from build123d import *

# Parameters (mm, degrees)
F1_DEPTH    = 20
F2_START    = 18.5
F2_DEPTH    = 1.5
F3_START    = 17.5
F0_W        = 1.9191285201
F0_H        = 0.8
F3_DEPTH    = 2
F4_START    = 17.5
F0_H_2      = 0.9897637812
F4_DEPTH    = 2
F5_DEPTH    = 17.5
F6_DEPTH    = 18.5
F7_START    = 17.5
F0_W_2      = 35
F0_H_3      = 9.3263725303
F7_DEPTH    = 2.5
F8_T1_DEPTH = 40.1796577476
F8_T3_DEPTH = 14.5060302779


# Not quite as in the source:
# - a fillet or chamfer that OpenCascade refuses, or shapes differently, is made with other operations: its cross-section is extruded or revolved along the edge and cut away or added


with BuildPart() as f1:
    # F0 (on Top) → F1 (new body)
    with BuildSketch(Plane.XY):
        Polygon((-14.85, 2), (14.85, 2), (14.85, -1), (14.85, -2), (0.95956426, -2), (0.95956426, -2.8), (15.65, -2.8), (15.65, 2.8), (-15.65, 2.8), (-15.65, -2.8), (-0.95956426, -2.8), (-0.95956426, -2), (-14.85, -2), (-14.85, -1), align=None)
    extrude(amount=F1_DEPTH)

    # F0 (on Top) → F2 (join)
    with BuildSketch(Plane.XY.offset(F2_START)):
        Polygon((14.85, -2), (14.85, -1), (-14.85, -1), (-14.85, -2), (-0.95956426, -2), (-0.95956426, -1.4462094987), (0.4121778399, -1.4462094987), (0.95956426, -2), align=None)
    extrude(amount=F2_DEPTH)

    # F0 (on Top) → F3 (join)
    with BuildSketch(Plane.XY.offset(F3_START)):
        with Locations((0, -2.4)):
            Rectangle(F0_W, F0_H)
        Polygon((-0.95956426, -2), (0.95956426, -2), (0.4121778399, -1.4462094987), (-0.95956426, -1.4462094987), align=None)
    extrude(amount=F3_DEPTH)

    # F0 (on Top) → F4 (join)
    with BuildSketch(Plane.XY.offset(F4_START)):
        with Locations((0, -3.2948818906)):
            Rectangle(F0_W, F0_H_2)
    extrude(amount=F4_DEPTH)

    # F0 (on Top) → F5 (join)
    with BuildSketch(Plane.XY):
        with Locations((0, -2.4)):
            Rectangle(F0_W, F0_H)
    extrude(amount=F5_DEPTH)

    # F0 (on Top) → F6 (cut)
    with BuildSketch(Plane.XY):
        Polygon((-0.95956426, -2), (0.95956426, -2), (0.4121778399, -1.4462094987), (-0.95956426, -1.4462094987), align=None)
    extrude(amount=F6_DEPTH, mode=Mode.SUBTRACT)

    # F0 (on Top) → F7 (join)
    with BuildSketch(Plane.XY.offset(F7_START)):
        with Locations((0, 0.4131862652)):
            Rectangle(F0_W_2, F0_H_3)
        Polygon((15.65, -2.8), (0.95956426, -2.8), (0.95956426, -3.7897637812), (-0.95956426, -3.7897637812), (-0.95956426, -2.8), (-15.65, -2.8), (-15.65, 2.8), (15.65, 2.8), align=None, mode=Mode.SUBTRACT)
    extrude(amount=F7_DEPTH)

    # F8: chamfer of 0.5 x 1 on 4 edges, made by hand

    # F8_s2 → F8_t1 (cut)
    with BuildSketch(Plane.YZ.offset(-20.0898288738)):
        Polygon((4.0763725303, 20), (5.0763725303, 19.5), (5.0763725303, 20), align=None)
        Polygon((-3.25, 20), (-4.25, 19.5), (-4.25, 20), align=None)
    extrude(amount=F8_T1_DEPTH, mode=Mode.SUBTRACT)

    # F8_s4 → F8_t3 (cut)
    with BuildSketch(Plane.XZ.offset(-7.6662014041)):
        Polygon((-17.5, 19.5), (-16.5, 20), (-17.5, 20), align=None)
        Polygon((16.5, 20), (17.5, 19.5), (17.5, 20), align=None)
    extrude(amount=F8_T3_DEPTH, mode=Mode.SUBTRACT)


solid = f1.part
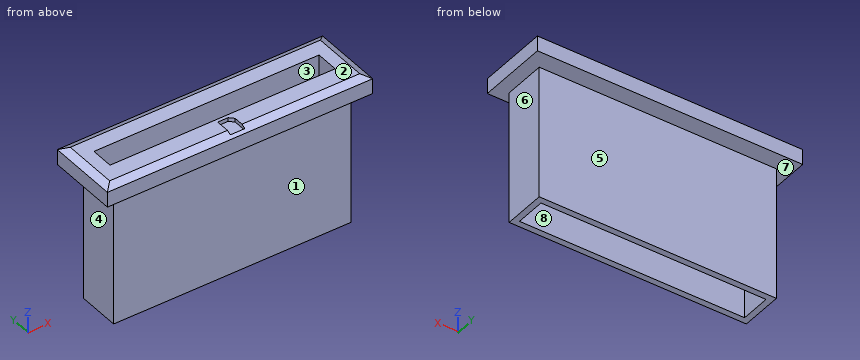
CAD build for the part. Positions are in the model's coordinates, mm. Face numbers are marked on the shaded views. A direction names the side the tool comes from. Round coordinates to 2 decimals unless told otherwise and drop trailing zeros. Write each loop counter-clockwise with the first axis right and the second up, starting at its lowest first coordinate (ties: lowest second). Pieces come first, ordered by that corner, then holes.
(1) Mould opens along X. For the marked faces 6, 7 and 8 say: pulls with the +X half, pulls with the -X half, needs draft (parallel to the pull), parting line crosses it, or undercut.
(2) Drop flat-ended pins along their axis: P1, Ø1.1, axis at x = -4.5, y = -1.5, coming from the -Z side; P2, Ø2, axis at y = 0, z = 12, coming from the +X side; P3, Ø1.5, axis at y = -3, z = 13.5, coming from the -X side; P4, Ø5.5, axis at x = 7, z = 6.5, coming from the +Y side. Give the stop position or say it passes through.
(3) 3-axis set-ups, long thin cutter, end or side, ignore diameter. For the marked faces 1, 2, 3, 4 and 5: which of +Z, -Z, +X, -X, +Y, -Y reach the whole face in a straight line?
(4) Slice it at C-C, the plane y = -0.5. Write the cut outline in (x, z).
(5) Slice it at B-B, the plane z = 6.5. Write the cut outline in (x, y), and give its area (3 significant figures).
(6) Slice it at A-A, the plane x = -0.5. Write the cut outline in (y, z).
(7) Probe line 1 along Y through (x, z) = (0, 4.75); line 2 along X through (y, z) = (0, 2.75); line 3 along Z through (x, y) = (12.5, -3). List the from-to ranges inside material, lowest first.
From the geometry:
1. face 6: pulls with the +X half
1. face 7: needs draft
1. face 8: undercut
2. P1: stops at z = 0
2. P2: stops at x = 15.65
2. P3: stops at x = -15.65
2. P4: stops at y = 2.8
3. face 1: -Z, +X, -X, -Y
3. face 2: +Z, +X, -X, +Y, -Y
3. face 3: +Z, -Z
3. face 4: -Z, -X, +Y, -Y
3. face 5: -Z, +X, -X, +Y
4. outline: (-17.5, 17.5) - (-15.65, 17.5) - (-15.65, 0) - (-14.85, 0) - (-14.85, 20) - (-16.5, 20) - (-17.5, 19.5) - close; (14.85, 0) - (15.65, 0) - (15.65, 17.5) - (17.5, 17.5) - (17.5, 19.5) - (16.5, 20) - (14.85, 20) - close
5. outline: (-15.65, -2.8) - (15.65, -2.8) - (15.65, 2.8) - (-15.65, 2.8) - close; hole (-14.85, -2) - (14.85, -2) - (14.85, 2) - (-14.85, 2) - close
5. area: 56.5 mm2
6. outline: (-4.25, 17.5) - (-2.8, 17.5) - (-2.8, 0) - (-2, 0) - (-2, 18.5) - (-1, 18.5) - (-1, 20) - (-1.45, 20) - (-1.45, 19.5) - (-3.79, 19.5) - (-3.79, 19.73) - (-4.25, 19.5) - close; (2, 0) - (2.8, 0) - (2.8, 17.5) - (5.08, 17.5) - (5.08, 19.5) - (4.08, 20) - (2, 20) - close
7. line 1: y = -2.8 to -2, 2 to 2.8
7. line 2: x = -15.65 to -14.85, 14.85 to 15.65
7. line 3: z = 17.5 to 20
